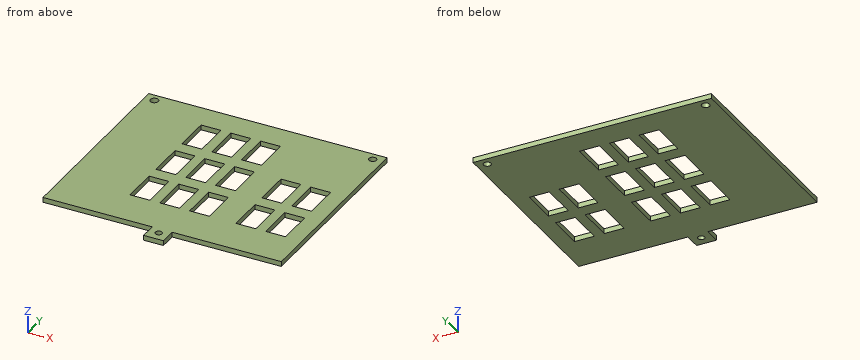
```python
from build123d import *

# Parameters (mm, degrees)
ESQUISSE1_W             = 72
ESQUISSE1_H             = 61
BOSS_EXTRU_1_DEPTH      = 1.5
ESQUISSE2_R             = 1.114499423
ESQUISSE2_R_2           = 1.207075002
ENL_V_MAT_EXTRU_1_DEPTH = 2.5
ESQUISSE4_W             = 6
ESQUISSE4_H             = 11
ENL_V_MAT_EXTRU_2_DEPTH = 2.5
ESQUISSE4_3_W           = 6
ESQUISSE4_3_H           = 11
ESQUISSE4_3_H_2         = 10.972423644
ENL_V_MAT_EXTRU_3_DEPTH = 2.5
ESQUISSE5_W             = 6
ESQUISSE5_H             = 1.5
BOSS_EXTRU_2_DEPTH      = 5
ESQUISSE6_R             = 1
ENL_V_MAT_EXTRU_4_DEPTH = 6


with BuildPart() as part:
    # Esquisse1 → Boss.-Extru.1 (new body)
    with BuildSketch(Plane.XY):
        with Locations((-31.584952854, -2.769073276)):
            Rectangle(ESQUISSE1_W, ESQUISSE1_H)
    extrude(amount=BOSS_EXTRU_1_DEPTH)

    # Esquisse2 → Enl_v. mat.-Extru.1 (cut, through all)
    with BuildSketch(Plane(origin=(0, 0, 0), x_dir=(-1, 0, 0), z_dir=(0, 0, -1))):
        with Locations((-1.415047146, 25.230926724)):
            Circle(ESQUISSE2_R)
        with Locations((64.584952854, 25.230926724)):
            Circle(ESQUISSE2_R_2)
    extrude(amount=-ENL_V_MAT_EXTRU_1_DEPTH, mode=Mode.SUBTRACT)

    # Esquisse4 → Enl_v. mat.-Extru.2 (cut, through all)
    with BuildSketch(Plane(origin=(0, 0, 0), x_dir=(-1, 0, 0), z_dir=(0, 0, -1))):
        with Locations((44.584952854, -15.769073276)):
            Rectangle(ESQUISSE4_W, ESQUISSE4_H)
        with Locations((35.584952854, -15.769073276)):
            Rectangle(ESQUISSE4_W, ESQUISSE4_H)
    extrude(amount=-ENL_V_MAT_EXTRU_2_DEPTH, mode=Mode.SUBTRACT)

    # Esquisse4_3 → Enl_v. mat.-Extru.3 (cut, through all)
    with BuildSketch(Plane(origin=(0, 0, 0), x_dir=(-1, 0, 0), z_dir=(0, 0, -1))):
        with Locations((26.584952854, -15.769073276)):
            Rectangle(ESQUISSE4_3_W, ESQUISSE4_3_H)
        with Locations((26.584952854, 14.230926724)):
            Rectangle(ESQUISSE4_3_W, ESQUISSE4_3_H)
        with Locations((44.584952854, -15.769073276)):
            Rectangle(ESQUISSE4_3_W, ESQUISSE4_3_H)
        with Locations((35.584952854, -15.769073276)):
            Rectangle(ESQUISSE4_3_W, ESQUISSE4_3_H)
        with Locations((44.584952854, -0.769073276)):
            Rectangle(ESQUISSE4_3_W, ESQUISSE4_3_H)
        with Locations((35.584952854, -0.782861454)):
            Rectangle(ESQUISSE4_3_W, ESQUISSE4_3_H_2)
        with Locations((26.584952854, -0.769073276)):
            Rectangle(ESQUISSE4_3_W, ESQUISSE4_3_H)
        with Locations((35.584952854, 14.203350368)):
            Rectangle(ESQUISSE4_3_W, ESQUISSE4_3_H)
        with Locations((44.584952854, 14.230926724)):
            Rectangle(ESQUISSE4_3_W, ESQUISSE4_3_H)
        with Locations((12.584952854, -15.769073276)):
            Rectangle(ESQUISSE4_3_W, ESQUISSE4_3_H)
        with Locations((3.584952854, -15.769073276)):
            Rectangle(ESQUISSE4_3_W, ESQUISSE4_3_H)
        with Locations((12.584952854, -0.769073276)):
            Rectangle(ESQUISSE4_3_W, ESQUISSE4_3_H)
        with Locations((3.584952854, -0.769073276)):
            Rectangle(ESQUISSE4_3_W, ESQUISSE4_3_H)
    extrude(amount=-ENL_V_MAT_EXTRU_3_DEPTH, mode=Mode.SUBTRACT)

    # Esquisse5 → Boss.-Extru.2 (add)
    with BuildSketch(Plane.XZ.offset(33.269073276)):
        with Locations((-31.584952854, 0.75)):
            Rectangle(ESQUISSE5_W, ESQUISSE5_H)
    extrude(amount=BOSS_EXTRU_2_DEPTH)

    # Esquisse6 → Enl_v. mat.-Extru.4 (cut)
    with BuildSketch(Plane.XY.offset(1.5)):
        with Locations((-31.584952854, -35.269073276)):
            Circle(ESQUISSE6_R)
    extrude(amount=-ENL_V_MAT_EXTRU_4_DEPTH, mode=Mode.SUBTRACT)


solid = part.part
```
Source: CAD feature listing. Evaluate the final solid. Frame: model axes, mm. Round coordinates to 2 decimals unless told otherwise and drop trailing zeros. Write each loop counter-clockwise with the first axis right and the second up, starting at its lowest first coordinate (ties: lowest second). Pieces come first, ordered by that corner, then holes. Notation, with made-up numbers: M -29.5,10.25 L -16.5,10.25 A11 cw -16.5,19.25 Z; hole C 30.25,71 d4. An arc over 180 degrees is marked long. Answer as a JSON object with one key per item and string values. Group by question number.
(1) Section query D-D on z = 0.9. State how many separate pieces and enclosed holes the cut face has, then the cut area to 3 significant figures.
(2) Section query A-A on y = 14.5. Output: boundary loops of the cut face in (x, z), then the cut area to 3 significant figures.
(3) Ray query, line 1 (X direction, y = -13.5, z = 0.35); line 2 (X direction, y = 11, z = 0.25); line 3 (Y direction, x = -13.5, z = 0.4). Return the intervals inside material, ascending. Write a range as [from, to].
(4) Section query B-B on x = -27.5. Output: boundary loops of the cut face in (y, z).
(5) Section query C-C on y = 3.5. Output: boundary loops of the cut face in (x, z).
Computed values:
{
 "1": {"separate pieces": "1", "enclosed holes": "16", "area": "3,550 mm^2"},
 "2": {"outline": "M -67.58,0 L -47.58,0 L -47.58,1.5 L -67.58,1.5 Z; M -41.58,0 L -38.58,0 L -38.58,1.5 L -41.58,1.5 Z; M -32.58,0 L -29.58,0 L -29.58,1.5 L -32.58,1.5 Z; M -23.58,0 L 4.42,0 L 4.42,1.5 L -23.58,1.5 Z", "area": "81.0 mm^2"},
 "3": {"line 1": "[-67.58, -47.58], [-41.58, -38.58], [-32.58, -29.58], [-23.58, -15.58], [-9.58, -6.58], [-0.58, 4.42]", "line 2": "[-67.58, -47.58], [-41.58, -38.58], [-32.58, -29.58], [-23.58, 4.42]", "line 3": "[-33.27, -21.27], [-10.27, -6.27], [4.73, 27.73]"},
 "4": {"outline": "M -33.27,0 L -21.27,0 L -21.27,1.5 L -33.27,1.5 Z; M -10.27,0 L -6.27,0 L -6.27,1.5 L -10.27,1.5 Z; M 4.73,0 L 8.73,0 L 8.73,1.5 L 4.73,1.5 Z; M 19.73,0 L 27.73,0 L 27.73,1.5 L 19.73,1.5 Z"},
 "5": {"outline": "M -67.58,0 L -47.58,0 L -47.58,1.5 L -67.58,1.5 Z; M -41.58,0 L -38.58,0 L -38.58,1.5 L -41.58,1.5 Z; M -32.58,0 L -29.58,0 L -29.58,1.5 L -32.58,1.5 Z; M -23.58,0 L -15.58,0 L -15.58,1.5 L -23.58,1.5 Z; M -9.58,0 L -6.58,0 L -6.58,1.5 L -9.58,1.5 Z; M -0.58,0 L 4.42,0 L 4.42,1.5 L -0.58,1.5 Z"}
}
